from build123d import *

# Parameters (mm, degrees)
BOSS_EXTRUDE1_DEPTH = 6
SKETCH2_R           = 3.429
CUT_EXTRUDE1_DEPTH  = 107.235587258
SKETCH3_R           = 9
CUT_EXTRUDE2_DEPTH  = 3
FILLET1_R           = 10


with BuildPart() as part:
    # Sketch1 → Boss-Extrude1 (new body)
    with BuildSketch(Plane.XY):
        Polygon((0, 0), (0, 75), (30, 75), (30, 30), (75, 30), (75, 0), align=None)
    extrude(amount=BOSS_EXTRUDE1_DEPTH)

    # Sketch2 → Cut-Extrude1 (cut, through all)
    with BuildSketch(Plane.XY.offset(6)):
        with Locations((15, 15)):
            Circle(SKETCH2_R)
        with Locations((15, 55.95)):
            Circle(SKETCH2_R)
        with Locations((55.95, 15)):
            Circle(SKETCH2_R)
    extrude(amount=-CUT_EXTRUDE1_DEPTH, mode=Mode.SUBTRACT)

    # Sketch3 → Cut-Extrude2 (cut)
    with BuildSketch(Plane.XY.offset(6)):
        with Locations((55.95, 15)):
            Circle(SKETCH3_R)
        with Locations((15, 15)):
            Circle(SKETCH3_R)
        with Locations((15, 55.95)):
            Circle(SKETCH3_R)
    extrude(amount=-CUT_EXTRUDE2_DEPTH, mode=Mode.SUBTRACT)

    # Fillet1
    fillet1_edges = [part.edges().sort_by_distance(p)[0] for p in [
        (0, 0, 3),
        (0, 75, 3),
        (30, 75, 3),
        (75, 30, 3),
        (75, 0, 3),
    ]]
    fillet(fillet1_edges, radius=FILLET1_R)


solid = part.part
Here's how the part is built. I have some questions about the finished solid (model axes, mm). A direction names the side the tool comes from. Give positions to 0.01 mm unless a question says otherwise; leave off trailing zeros. Order: outer loops, then holes, each group sorted by start corner. A loop starts at its lowest first (then second) coordinate and runs counter-clockwise, first axis right, second up. Notation, with made-up numbers: (-27.75, 71) -> (12.25, 71) arc R27 cw to (12.25, 97) -> close; hole circle Ø10 at (11, 62). An arc over 180 degrees is marked (long way). Use a Markdown table: item, result. Add a question column.
Item 1: I need wall thicknesses on line 1 (Y direction, x = 15, z = 3.9); line 2 (Y direction, x = 15, z = 0.75); line 3 (Y direction, x = 31, z = 4.35). Which ranges of each line are inside material? Lowest first, please.
Item 2: If we mould it in two halves opening along X, with no side actions, what happens to faces 1 (the face through (15, 11, 3)), 2 (the face through (12.28, 53.86, 1.52)), 3 (the face through (71.99, 2.85, 3.04)), 4 (the face through (0, 37, 3))? For each: pulls with the +X half, pulls with the -X half, needs draft (parallel to the pull), parting line crosses it, or undercut.
Item 3: For faces 5 (the face through (15, 75, 3)), 6 (the face through (47, 30, 3)), 7 (the face through (64.534, 17.703, 4.521)), which set-ups out of +Z, -Z, +X, -X, +Y, -Y let a thin tool reach every point of the face, with its end or its side?
Item 4: Imagine slicing it at D-D on z = 4.1. Please give me the cut outline in (x, y).
Item 5: Imagine slicing it at B-B on x = 55.95. Please give me the cut outline in (y, z), plus the area to 3 significant figures.
Item 6: Will these pins go through, and if not, where does the flat tip stop? pin 1 (11 mm diameter, centred on x = 55.95, y = 15, fed in from +Z); pin 2 (2 mm diameter, centred on x = 46.5, z = 1.5, fed in from +Y); pin 3 (1.5 mm diameter, centred on y = 32, z = 4.5, fed in from +X).
Item 7: Imagine slicing it at A-A on y = 15. Please give me the cut outline in (x, z), plus the area to 3 significant figures.
Data:
| question | item | result |
|---|---|---|
| 1 | line 1 | y = 0 to 6, 24 to 46.95, 64.95 to 75 |
| 1 | line 2 | y = 0 to 11.57, 18.43 to 52.52, 59.38 to 75 |
| 1 | line 3 | y = 0 to 30 |
| 2 | face 1 | undercut |
| 2 | face 2 | undercut |
| 2 | face 3 | pulls with the +X half |
| 2 | face 4 | pulls with the -X half |
| 3 | face 5 | +Z, -Z, +X, -X, +Y |
| 3 | face 6 | +Z, -Z, +X, +Y |
| 3 | face 7 | +Z |
| 4 | outline | (0, 10) arc R10 ccw to (10, 0) -> (65, 0) arc R10 ccw to (75, 10) -> (75, 20) arc R10 ccw to (65, 30) -> (30, 30) -> (30, 65) arc R10 ccw to (20, 75) -> (10, 75) arc R10 ccw to (0, 65) -> close; hole circle Ø18 at (15, 15); hole circle Ø18 at (15, 55.95); hole circle Ø18 at (55.95, 15) |
| 5 | outline | (0, 0) -> (11.57, 0) -> (11.57, 3) -> (6, 3) -> (6, 6) -> (0, 6) -> close; (18.43, 0) -> (30, 0) -> (30, 6) -> (24, 6) -> (24, 3) -> (18.43, 3) -> close |
| 5 | area | 105 mm² |
| 6 | pin 1 | stops at z = 3 |
| 6 | pin 2 | stops at y = 30 |
| 6 | pin 3 | stops at x = 30 |
| 7 | outline | (0, 0) -> (11.57, 0) -> (11.57, 3) -> (6, 3) -> (6, 6) -> (0, 6) -> close; (18.43, 0) -> (52.52, 0) -> (52.52, 3) -> (46.95, 3) -> (46.95, 6) -> (24, 6) -> (24, 3) -> (18.43, 3) -> close; (59.38, 0) -> (75, 0) -> (75, 6) -> (64.95, 6) -> (64.95, 3) -> (59.38, 3) -> close |
| 7 | area | 301 mm² |
